Geometry: final body of the model. Coordinates: model frame, mm. A direction names the side the tool comes from. Give positions to 0.01 mm unless a question says otherwise; leave off trailing zeros. Write each loop counter-clockwise with the first axis right and the second up, starting at its lowest first coordinate (ties: lowest second). Pieces come first, ordered by that corner, then holes.
from build123d import *

# Parameters (mm, degrees)
F0_R     = 3.1
F1_DEPTH = 1
F2_DEPTH = 5.3
F3_R     = 7.282243


with BuildPart() as f1:
    # F0 (on Top) → F1 (new body)
    with BuildSketch(Plane.XY):
        with BuildLine():
            Line((-12.504604, -5.433536), (-53.033009, -45.961941))
            ThreePointArc((-53.033009, -45.961941), (-53.033009, -53.033009), (-45.961941, -53.033009))
            Line((-45.961941, -53.033009), (-5.428932, -12.5))
            Line((-5.428932, -12.5), (-5.35066, -12.421728))
            Line((-5.35066, -12.421728), (12.495396, -12.421728))
            Line((12.495396, -12.421728), (12.495396, 12.5))
            Line((12.495396, 12.5), (-12.5, 12.5))
            Line((-12.5, 12.5), (-12.5, -5.428932))
            Line((-12.5, -5.428932), (-12.504604, -5.433536))
        make_face()
        with BuildLine():
            Line((-8.854604, 7.328272), (-7.254604, 8.928272))
            Line((-7.254604, 8.928272), (-3.854604, 8.928272))
            ThreePointArc((-3.854604, 8.928272), (-0.004604, 7.328272), (3.845396, 8.928272))
            Line((3.845396, 8.928272), (7.245396, 8.928272))
            Line((7.245396, 8.928272), (8.845396, 7.328272))
            Line((8.845396, 7.328272), (8.845396, 3.928272))
            ThreePointArc((8.845396, 3.928272), (7.245396, 0.078272), (8.845396, -3.771728))
            Line((8.845396, -3.771728), (8.845396, -7.171728))
            Line((8.845396, -7.171728), (7.245396, -8.771728))
            Line((7.245396, -8.771728), (3.845396, -8.771728))
            ThreePointArc((3.845396, -8.771728), (-0.004604, -7.171728), (-3.854604, -8.771728))
            Line((-3.854604, -8.771728), (-7.254604, -8.771728))
            Line((-7.254604, -8.771728), (-8.854604, -7.171728))
            Line((-8.854604, -7.171728), (-8.854604, -3.771728))
            ThreePointArc((-8.854604, -3.771728), (-7.254604, 0.078272), (-8.854604, 3.928272))
            Line((-8.854604, 3.928272), (-8.854604, 7.328272))
        make_face(mode=Mode.SUBTRACT)
        with BuildLine():
            Line((-3.854604, 8.928272), (-7.254604, 8.928272))
            Line((-7.254604, 8.928272), (-8.854604, 7.328272))
            Line((-8.854604, 7.328272), (-8.854604, 3.928272))
            ThreePointArc((-8.854604, 3.928272), (-7.254604, 0.078272), (-8.854604, -3.771728))
            Line((-8.854604, -3.771728), (-8.854604, -7.171728))
            Line((-8.854604, -7.171728), (-7.254604, -8.771728))
            Line((-7.254604, -8.771728), (-3.854604, -8.771728))
            ThreePointArc((-3.854604, -8.771728), (-0.004604, -7.171728), (3.845396, -8.771728))
            Line((3.845396, -8.771728), (7.245396, -8.771728))
            Line((7.245396, -8.771728), (8.845396, -7.171728))
            Line((8.845396, -7.171728), (8.845396, -3.771728))
            ThreePointArc((8.845396, -3.771728), (7.245396, 0.078272), (8.845396, 3.928272))
            Line((8.845396, 3.928272), (8.845396, 7.328272))
            Line((8.845396, 7.328272), (7.245396, 8.928272))
            Line((7.245396, 8.928272), (3.845396, 8.928272))
            ThreePointArc((3.845396, 8.928272), (-0.004604, 7.328272), (-3.854604, 8.928272))
        make_face()
        with Locations((-0.004604, 0.078272)):
            Circle(F0_R, mode=Mode.SUBTRACT)
        with Locations((-0.004604, 0.078272)):
            Circle(F0_R)
    extrude(amount=-F1_DEPTH)

    # F0 (on Top) → F2 (join)
    with BuildSketch(Plane.XY):
        with BuildLine():
            Line((-12.504604, -5.433536), (-53.033009, -45.961941))
            ThreePointArc((-53.033009, -45.961941), (-53.033009, -53.033009), (-45.961941, -53.033009))
            Line((-45.961941, -53.033009), (-5.428932, -12.5))
            Line((-5.428932, -12.5), (-5.35066, -12.421728))
            Line((-5.35066, -12.421728), (12.495396, -12.421728))
            Line((12.495396, -12.421728), (12.495396, 12.5))
            Line((12.495396, 12.5), (-12.5, 12.5))
            Line((-12.5, 12.5), (-12.5, -5.428932))
            Line((-12.5, -5.428932), (-12.504604, -5.433536))
        make_face()
        with BuildLine():
            Line((-8.854604, 7.328272), (-7.254604, 8.928272))
            Line((-7.254604, 8.928272), (-3.854604, 8.928272))
            ThreePointArc((-3.854604, 8.928272), (-0.004604, 7.328272), (3.845396, 8.928272))
            Line((3.845396, 8.928272), (7.245396, 8.928272))
            Line((7.245396, 8.928272), (8.845396, 7.328272))
            Line((8.845396, 7.328272), (8.845396, 3.928272))
            ThreePointArc((8.845396, 3.928272), (7.245396, 0.078272), (8.845396, -3.771728))
            Line((8.845396, -3.771728), (8.845396, -7.171728))
            Line((8.845396, -7.171728), (7.245396, -8.771728))
            Line((7.245396, -8.771728), (3.845396, -8.771728))
            ThreePointArc((3.845396, -8.771728), (-0.004604, -7.171728), (-3.854604, -8.771728))
            Line((-3.854604, -8.771728), (-7.254604, -8.771728))
            Line((-7.254604, -8.771728), (-8.854604, -7.171728))
            Line((-8.854604, -7.171728), (-8.854604, -3.771728))
            ThreePointArc((-8.854604, -3.771728), (-7.254604, 0.078272), (-8.854604, 3.928272))
            Line((-8.854604, 3.928272), (-8.854604, 7.328272))
        make_face(mode=Mode.SUBTRACT)
        with Locations((-0.004604, 0.078272)):
            Circle(F0_R)
    extrude(amount=F2_DEPTH)

    # F3
    f3_edges = [f1.edges().sort_by_distance(p)[0] for p in [
        (-12.5, -5.428932, 2.15),
        (-12.5, 12.5, 2.15),
        (12.495396, 12.5, 2.15),
        (12.495396, -12.421728, 2.15),
        (-5.35066, -12.421728, 2.15),
    ]]
    fillet(f3_edges, radius=F3_R)


solid = f1.part
Q1. Pull-direction query (Y, two-part tool) for faces 4 (the flat face through (-21, -21, 5.3)), 5 (the cylindrical face through (-7.255, 0.018, 2.613)), 6 (the cylindrical face through (-5.08, -12.96, 2.19)); classes: released by +Y, released by -Y, zero draft, split by the parting line, or undercut.
Filled sheet:
face 4: zero draft
face 5: undercut
face 6: released by -Y
Q2. Access query for faces 1 (the cylindrical face through (2.95, 1.01, 2.61)), 2 (the cylindrical face through (-10.423, 10.31, 2.106)), 3 (the flat face through (1, -12.422, 2)). Directions: +Z, -Z, +X, -X, +Y, -Y. A direction counts if a zero-diameter tool reaches every point of the face in a straight line with its end or side. Return the directions, or none.
Filled sheet:
face 1: +Z
face 2: +Z, -Z, -X, +Y
face 3: +Z, -Z, +X, -Y
Q3. Section A-A on z = 3.25. Count the separate pieces of the cut face and the enclosed holes in it, plus the area to 3 significant figures.
Filled sheet:
separate pieces: 2
enclosed holes: 1
area: 935 mm2
Q4. Section C-C on y = -18.5. Output: boundary loops of the cut face in (x, z), plus the area to 3 significant figures.
Filled sheet:
outline: (-25.57, -1) - (-11.43, -1) - (-11.43, 5.3) - (-25.57, 5.3) - close
area: 89.1 mm2
Q5. Section B-B on x = -1.5. Output: boundary loops of the cut face in (y, z).
Filled sheet:
outline: (-12.42, -1) - (12.5, -1) - (12.5, 5.3) - (7.54, 5.3) - (7.54, 0) - (2.79, 0) - (2.79, 5.3) - (-2.64, 5.3) - (-2.64, 0) - (-7.38, 0) - (-7.38, 5.3) - (-12.42, 5.3) - close
Q6. Pin query (flat end, axial travel): P1, Ø1.7, axis at x = -6, z = 1.5, coming from the -Y side; P2, Ø1, axis at y = 6.5, z = 2.5, coming from the +X side; P3, Ø2.5, axis at x = 5.5, z = 3.5, coming from the -Y side. Return the tip coordinate at first contact, or that it passes through.
Filled sheet:
P1: stops at y = -13.99
P2: stops at x = 12.45
P3: stops at y = -12.42
Q7. Section D-D on x = -48. Output: boundary loops of the cut face in (y, z).
Filled sheet:
outline: (-54.27, -1) - (-40.93, -1) - (-40.93, 5.3) - (-54.27, 5.3) - close
Q8. Ray query, line 1 along Y through (x, z) = (0, 1.75); line 2 along Z through (x, y) = (5.5, 8); line 3 along Y through (x, z) = (5.5, 3.25). Return the intervals inside material, ascending.
Filled sheet:
line 1: y = -12.42 to -7.17, -3.02 to 3.18, 7.33 to 12.5
line 2: z = -1 to 0
line 3: y = -12.42 to -8.77, 8.93 to 12.49
